from build123d import *

# Parameters (mm, degrees)
BOSS_EXTRUDE1_DEPTH = 300
SKETCH2_W           = 600
SKETCH2_H           = 100
CUT_EXTRUDE1_DEPTH  = 250


with BuildPart() as part:
    # Sketch1 → Boss-Extrude1 (new body)
    with BuildSketch(Plane.XY):
        Polygon((-300, 400), (-300, 0), (300, 0), (-100, 400), align=None)
    boss_extrude1 = extrude(amount=BOSS_EXTRUDE1_DEPTH)

    # Sketch2 → Cut-Extrude1 (cut)
    with BuildSketch(Plane(origin=(0, 400, 0), x_dir=(1, 0, 0), z_dir=(0, 1, 0))):
        with Locations((0, -50)):
            Rectangle(SKETCH2_W, SKETCH2_H)
    cut_extrude1 = extrude(amount=-CUT_EXTRUDE1_DEPTH, mode=Mode.SUBTRACT)

    # Mirror1: Boss-Extrude1, Cut-Extrude1 across plane
    add(boss_extrude1.mirror(Plane.XY))
    add(cut_extrude1.mirror(Plane.XY), mode=Mode.SUBTRACT)


solid = part.part
The listing builds one solid part. Answer for the finished solid, in the listing's coordinates (mm). A direction names the side the tool comes from. Coordinates: 2 decimals unless noted, no trailing zeros. Write each loop counter-clockwise with the first axis right and the second up, starting at its lowest first coordinate (ties: lowest second). Pieces come first, ordered by that corner, then holes. Notation, with made-up numbers: (41, -22) - (66, -22) arc R21 ccw to (66, -14) - close; hole circle Ø6 at (21.5, -7.75). An arc over 180 degrees is marked (long way). Put each result on its own line as item: value.
1. Find the intervals of material crossed by line 1 along Z through (x, y) = (-48, 295.5); line 2 along Y through (x, z) = (-106.5, -60.5); line 3 along Y through (x, z) = (91, 117), in increasing order. Write a range as from..to.
Answer sheet:
line 1: z = -300..-100, 100..300
line 2: y = 0..150
line 3: y = 0..209
2. Determine the mould class of faces 3 (the face through (-78, 150, 1)), 4 (the face through (-71, 158, -300)), 5 (the face through (-300, 114, 4)) for opening direction Z: pulls with the +Z half, pulls with the -Z half, needs draft (parallel to the pull), parting line crosses it, or undercut.
Answer sheet:
face 3: undercut
face 4: pulls with the -Z half
face 5: needs draft
3. The part is cut by section A-A on y = 334. Give the vertices of the cut face in (x, z).
Answer sheet:
outline: (-300, -300) - (-34, -300) - (-34, -100) - (-300, -100) - close; (-300, 100) - (-34, 100) - (-34, 300) - (-300, 300) - close
4. The part is cut by section C-C on y = 194. Give the vertices of the cut face in (x, z).
Answer sheet:
outline: (-300, -300) - (106, -300) - (106, -100) - (-300, -100) - close; (-300, 100) - (106, 100) - (106, 300) - (-300, 300) - close
5. The part is cut by section B-B on x = -261. Give the vertices of the cut face in (y, z), plus the area to 3 significant figures.
Answer sheet:
outline: (0, -300) - (400, -300) - (400, -100) - (150, -100) - (150, 100) - (400, 100) - (400, 300) - (0, 300) - close
area: 190,000 mm^2
6. Flat-ended cylindrical pins translate along their axes: pin 1 Ø10 at (y, z) = (152, 27.5) entering from +X; pin 2 Ø12 at (x, z) = (193.5, 13) entering from +Y; pin 3 Ø6 at (y, z) = (193.5, 163) entering from +X. Find the tip coordinate at first contact, or state that the pin passes through.
Answer sheet:
pin 1: stops at x = 153
pin 2: stops at y = 112.5
pin 3: stops at x = 109.5
7. A tool of negligible diameter and unlimited length cuts with its end or side. For faces 1 (the face through (-4, 0, 4)), 2 (the face through (-128, 249, 100)), from which of +Z, -Z, +X, -X, +Y, -Y can it reach the whole face along a straight path? Write none if from no direction.
Answer sheet:
face 1: +Z, -Z, +X, -X, -Y
face 2: +X, -X, +Y
8. The part is cut by section D-D on z = -222.5. Give the vertices of the cut face in (x, y), plus the area to 3 significant figures.
Answer sheet:
outline: (-300, 0) - (300, 0) - (-100, 400) - (-300, 400) - close
area: 160,000 mm^2
